Verification items for this drawing (mm, ordinates from the low corner). A direction names the side the tool comes from. Round coordinates to 2 decimals unless told otherwise and drop trailing zeros. Write each loop counter-clockwise with the first axis right and the second up, starting at its lowest first coordinate (ties: lowest second). Pieces come first, ordered by that corner, then holes. Notation, with made-up numbers: (-30, 70.5) -> (-6, 70.5) arc R21 ccw to (-6, 101.5) -> close; hole circle Ø10 at (-16.75, 85.25). An arc over 180 degrees is marked (long way). One line per item, written item: value.
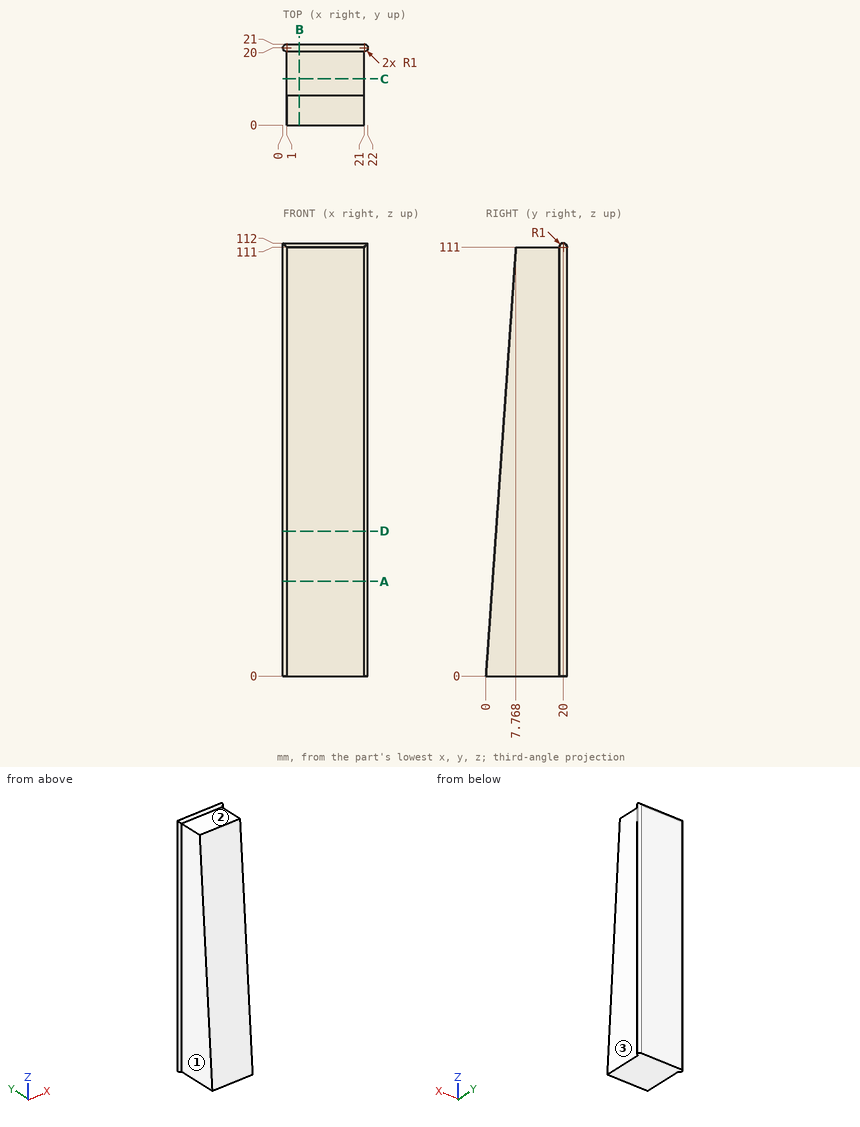
Item 1: Tool access check on the marked faces 1, 2 and 3. Record the directions out of +Z, -Z, +X, -X, +Y, -Y that give a thin tool (end or side, any length) a straight path to the whole face; none if there is none.
Result set:
face 1: +Z, -Z, -X, -Y
face 2: +Z, +X, -X, -Y
face 3: +Z, -Z, +X, -Y
Item 2: Sectioned sample at A-A (z = 24.5). Enter the section's corners in (x, y) (1 decimal), then the cut area to 3 significant figures.
Result set:
outline: (1, 1.7) -> (21, 1.7) -> (21, 19) arc R1 ccw to (21, 21) -> (1, 21) arc R1 ccw to (1, 19) -> close
area: 389 mm^2
Item 3: Depth check by flat-ended pin: pin 1 (9.5 mm diameter, centred on y = 14, z = 63, fed in from -X); pin 2 (4 mm diameter, centred on y = 10.5, z = 59.5, fed in from +X); pin 3 (3 mm diameter, centred on x = 11.5, y = 9.5, fed in from +Z). Enter the tip coordinate at first touch or a pass-through.
Result set:
pin 1: x = 1
pin 2: x = 21
pin 3: z = 111
Item 4: Sectioned sample at D-D (z = 37.5). Enter the section's corners in (x, y).
Result set:
outline: (1, 2.62) -> (21, 2.62) -> (21, 19) arc R1 ccw to (21, 21) -> (1, 21) arc R1 ccw to (1, 19) -> close
Item 5: Sectioned sample at C-C (y = 12). Enter the section's corners in (x, z).
Result set:
outline: (1, 0) -> (21, 0) -> (21, 111) -> (1, 111) -> close
Item 6: Material ranges on line 1 along X through (y, z) = (11.5, 6); line 2 along Z through (x, y) = (6, 13); line 3 along Y through (x, z) = (3.5, 81), recorded low to high.
Result set:
line 1: 1 to 21
line 2: 0 to 111
line 3: 5.67 to 21
Item 7: Sectioned sample at B-B (x = 4.25). Enter the section's corners in (y, z).
Result set:
outline: (0, 0) -> (21, 0) -> (21, 111) arc R1 ccw to (19, 111) -> (7.77, 111) -> close
